```python
from build123d import *

# Parameters (mm, degrees)
SKETCH1_W           = 105.41
SKETCH1_H           = 82
SKETCH1_R           = 1.0795
SKETCH1_R_2         = 1.27
BOSS_EXTRUDE1_DEPTH = 1.778
BOSS_EXTRUDE2_DEPTH = 0.2


with BuildPart() as part:
    # Sketch1 → Boss-Extrude1 (new body)
    with BuildSketch(Plane.XY):
        Rectangle(SKETCH1_W, SKETCH1_H)
        with Locations((46.482, 12.7)):
            Circle(SKETCH1_R, mode=Mode.SUBTRACT)
        with Locations((46.482, -12.7)):
            Circle(SKETCH1_R, mode=Mode.SUBTRACT)
        with Locations((-46.482, 12.7)):
            Circle(SKETCH1_R, mode=Mode.SUBTRACT)
        with Locations((-46.482, -12.7)):
            Circle(SKETCH1_R, mode=Mode.SUBTRACT)
        with Locations((-46.482, -19.05)):
            Circle(SKETCH1_R_2, mode=Mode.SUBTRACT)
    extrude(amount=BOSS_EXTRUDE1_DEPTH)

    # Sketch2 → Boss-Extrude2 (add)
    with BuildSketch(Plane.XY.offset(1.778)):
        Polygon((-9.175, 39.095), (0.825, 29.095), (0.825, -29.095), (-9.175, -39.095), (-42.705, -39.095), (-42.705, 39.095), align=None)
        Polygon((46.355, 20.205), (42.545, 16.395), (42.545, -16.395), (46.355, -20.205), (46.355, -29.095), (36.355, -39.095), (2.825, -39.095), (2.825, 39.095), (36.355, 39.095), (46.355, 29.095), align=None)
    extrude(amount=BOSS_EXTRUDE2_DEPTH)


solid = part.part
```
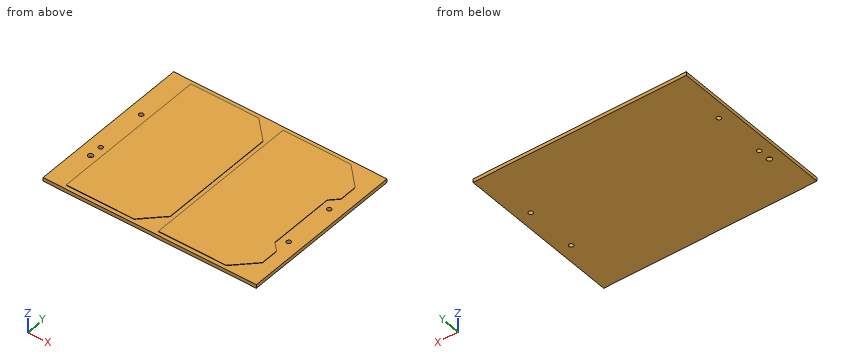
The model under review builds one solid part; all positions refer to its coordinate system, in mm. Give positions to 0.01 mm unless a question says otherwise; leave off trailing zeros. Write each loop counter-clockwise with the first axis right and the second up, starting at its lowest first coordinate (ties: lowest second). Pieces come first, ordered by that corner, then holes. Notation, with made-up numbers: (-17.75, 39) -> (35.25, 39) arc R25 cw to (35.25, 66) -> close; hole circle Ø9 at (23, 75.5). An arc over 180 degrees is marked (long way). Put each result on its own line as item: value.
(1) To check wall thickness, follow probe 1 along Z at (x, y) = (2, 17). State the ranges of the line that lie inside material, in increasing order. Write a range as from..to.
Results are:
probe 1: 0..1.78
(2) We need section C-C, the plane y = -33. Give the boundary of the cut face in (x, z) (3 decimals), and give its area (3 significant figures).
Results are:
outline: (-52.705, 0) -> (52.705, 0) -> (52.705, 1.778) -> (42.45, 1.778) -> (42.45, 1.978) -> (2.825, 1.978) -> (2.825, 1.778) -> (-3.08, 1.778) -> (-3.08, 1.978) -> (-42.705, 1.978) -> (-42.705, 1.778) -> (-52.705, 1.778) -> close
area: 203 mm²
(3) For pin 1 Ø2.5 at (x, y) = (-46.482, 12.7) entering from +Z, flat-tipped, find the tip position at first contact; note if it passes through.
Results are:
pin 1: z = 1.78
(4) We need section A-A, the plane y = 12.7. State how many separate pieces and enclosed holes the cut face has, and give its area (3 significant figures).
Results are:
separate pieces: 3
enclosed holes: 0
area: 196 mm²
(5) We need section B-B, the plane y = -19.05. Give the boundary of the cut face in (x, z) (3 decimals).
Results are:
outline: (-52.705, 0) -> (-47.752, 0) -> (-47.752, 1.778) -> (-52.705, 1.778) -> close; (-45.212, 0) -> (52.705, 0) -> (52.705, 1.778) -> (45.2, 1.778) -> (45.2, 1.978) -> (2.825, 1.978) -> (2.825, 1.778) -> (0.825, 1.778) -> (0.825, 1.978) -> (-42.705, 1.978) -> (-42.705, 1.778) -> (-45.212, 1.778) -> close
